from build123d import *

# Parameters (mm, degrees)
F0_W          = 30
F0_H          = 10
F1_DEPTH      = 2
F0_H_2        = 2.5
F2_DEPTH      = 8
F3_R          = 2.75
F3_R_2        = 2
F4_DEPTH      = 25
F4_DEPTH_BACK = 25


with BuildPart() as f1:
    # F0 (on Top) → F1 (new body)
    with BuildSketch(Plane.XY):
        Rectangle(F0_W, F0_H)
    extrude(amount=F1_DEPTH)

    # F0 (on Top) → F2 (join)
    with BuildSketch(Plane.XY):
        with Locations((0, -6.25)):
            Rectangle(F0_W, F0_H_2)
        Rectangle(F0_W, F0_H)
        with Locations((0, 6.25)):
            Rectangle(F0_W, F0_H_2)
    extrude(amount=-F2_DEPTH)

    # F3 (on Top) → F4 (cut, two sides)
    with BuildSketch(Plane.XY) as f4_sk:
        with Locations((-7.5, 0)):
            Circle(F3_R)
        with Locations((7.5, 0)):
            Circle(F3_R_2)
    extrude(amount=F4_DEPTH, mode=Mode.SUBTRACT)
    extrude(f4_sk.sketch, amount=-F4_DEPTH_BACK, mode=Mode.SUBTRACT)


solid = f1.part
Geometry: final body of the model. Coordinates: model frame, mm. A direction names the side the tool comes from. Round coordinates to 2 decimals unless told otherwise and drop trailing zeros. Loops run counter-clockwise (first coordinate to the right, second up) from the corner with the lowest first, then second, coordinate; pieces in that order, holes last. Notation, with made-up numbers: M -37.75,62.5 L 19.25,62.5 A25 ccw 19.25,81.5 Z; hole C 77.25,50 d6. An arc over 180 degrees is marked long. Put each result on its own line as item: value. Start each with the question number.
(1) Set-up query: faces 5 (the face through (0, 0, 2)), 6 (the face through (0, -6, 0)), 7 (the face through (0, 5, 1)). Return all of +Z, -Z, +X, -X, +Y, -Y with unobstructed straight access to the full face (end or side cutting, diameter ignored); none if empty.
(2) Section query B-B (x = 7.5). Return loops of the section in (y, z), then the cut area to 3 significant figures.
(3) Section query C-C (z = -1). Return loops of the section in (x, y), then the cut area to 3 significant figures.
(4) Draft query along X for faces 1 (the face through (0, -5, 1)), 2 (the face through (15, 0, -3)), 3 (the face through (5.502, 0.088, -2.93)), 4 (the face through (-15, 0, -3)). Return one class per face: +X half, -X half, draft (parallel to the pull), parting line (faces both ways), or undercut.
(5) Material intervals for line 1 along X through (y, z) = (0, -1.5); line 2 along X through (y, z) = (1.25, 1.25); line 3 along Y through (x, z) = (7.5, -6), sorted ascending. Write a range as [from, to].
(6) Contact query for a flat-ended pin moving along its axis: pin 1 Ø0.6 at (x, z) = (2.5, 0.5) entering from +Y. Output: stop coordinate, or through.
(7) Section query A-A (y = 0). Return loops of the section in (x, z), then the cut area to 3 significant figures.
(8) Section query D-D (x = -7.5). Return loops of the section in (y, z), then the cut area to 3 significant figures.
Findings below:
1. face 5: +Z, +X, -X, +Y, -Y
1. face 6: +Z, +X, -X, -Y
1. face 7: +Z, +X, -X, +Y
2. outline: M -7.5,-8 L -2,-8 L -2,2 L -5,2 L -5,0 L -7.5,0 Z; M 2,-8 L 7.5,-8 L 7.5,0 L 5,0 L 5,2 L 2,2 Z
2. area: 100 mm2
3. outline: M -15,-7.5 L 15,-7.5 L 15,7.5 L -15,7.5 Z; hole C -7.5,0 d5.5; hole C 7.5,0 d4
3. area: 414 mm2
4. face 1: draft
4. face 2: +X half
4. face 3: undercut
4. face 4: -X half
5. line 1: x = [-15, -10.25], [-4.75, 5.5], [9.5, 15]
5. line 2: x = [-15, -9.95], [-5.05, 5.94], [9.06, 15]
5. line 3: y = [-7.5, -2], [2, 7.5]
6. pin 1: stops at y = 5
7. outline: M -15,-8 L -10.25,-8 L -10.25,2 L -15,2 Z; M -4.75,-8 L 5.5,-8 L 5.5,2 L -4.75,2 Z; M 9.5,-8 L 15,-8 L 15,2 L 9.5,2 Z
7. area: 205 mm2
8. outline: M -7.5,-8 L -2.75,-8 L -2.75,2 L -5,2 L -5,0 L -7.5,0 Z; M 2.75,-8 L 7.5,-8 L 7.5,0 L 5,0 L 5,2 L 2.75,2 Z
8. area: 85.0 mm2
